Input: part model. Units: mm. Frame: model coordinates. A direction names the side the tool comes from. Coordinates: 2 decimals unless noted, no trailing zeros. Loops run counter-clockwise (first coordinate to the right, second up) from the corner with the lowest first, then second, coordinate; pieces in that order, holes last. Notation, with made-up numbers: (-26.5, 62) - (-7.5, 62) arc R15 ccw to (-7.5, 84) - close; hole circle Ø4 at (47, 89.5). An arc over 180 degrees is marked (long way). Use one line per item in the form item = value.
from build123d import *

# Parameters (mm, degrees)
F0_W     = 510
F0_H     = 1610
F1_DEPTH = 18
F2_R     = 17.5
F3_DEPTH = 12


with BuildPart() as f1:
    # F0 (on Front) → F1 (new body)
    with BuildSketch(Plane.XZ):
        Rectangle(F0_W, F0_H)
    extrude(amount=F1_DEPTH)

    # F2 (on face) → F3 (cut)
    with BuildSketch(Plane(origin=(0, 0, 0), x_dir=(-1, 0, 0), z_dir=(0, 1, 0))):
        with Locations((233.5, -755)):
            Circle(F2_R)
        with Locations((233.5, 0)):
            Circle(F2_R)
        with Locations((233.5, 755)):
            Circle(F2_R)
    extrude(amount=-F3_DEPTH, mode=Mode.SUBTRACT)


solid = f1.part
Q1. First-contact query: P1, Ø10.5, axis at x = -226, z = 751.5, coming from the +Y side. Flat tip, straight axial feed; report the tip coordinate or a pass-through.
Check values:
P1 = -12
Q2. Cut plane B-B, the plane x = -233.5. Return loops of the section in (y, z), then the cut area to 3 significant figures.
Check values:
outline = (-18, -805) - (0, -805) - (0, -772.5) - (-12, -772.5) - (-12, -737.5) - (0, -737.5) - (0, -17.5) - (-12, -17.5) - (-12, 17.5) - (0, 17.5) - (0, 737.5) - (-12, 737.5) - (-12, 772.5) - (0, 772.5) - (0, 805) - (-18, 805) - close
area = 27,700 mm²
Q3. Set-up query: faces 4 (the flat face through (-4, -18, 11)), 5 (the flat face through (-233, -12, -755)). Return all of +Z, -Z, +X, -X, +Y, -Y with unobstructed straight access to the full face (end or side cutting, diameter ignored); none if empty.
Check values:
face_4 = +Z, -Z, +X, -X, -Y
face_5 = +Y
Q4. Pull-direction query (Z, two-part tool) for faces 1 (the cylindrical face through (-216.017, -5.916, -754.231)), 2 (the flat face through (-4, 0, 11)), 3 (the flat face through (-233, -12, 755)); classes: pulls with the +Z half, pulls with the -Z half, needs draft (parallel to the pull), parting line crosses it, or undercut.
Check values:
face_1 = undercut
face_2 = needs draft
face_3 = undercut
Q5. Cut plane A-A, the plane z = 0. Return loops of the section in (x, y).
Check values:
outline = (-255, -18) - (255, -18) - (255, 0) - (-216, 0) - (-216, -12) - (-251, -12) - (-251, 0) - (-255, 0) - close
Q6. Ray query, line 1 along Z through (x, y) = (-233.5, -8.75). Return the intervals inside material, ascending. Write a range as [from, to].
Check values:
line_1 = [-805, -772.5], [-737.5, -17.5], [17.5, 737.5], [772.5, 805]
